The model under review builds one solid part; all positions refer to its coordinate system, in mm. Face numbers are marked on the shaded views. A direction names the side the tool comes from. Give positions to 0.01 mm unless a question says otherwise; leave off trailing zeros. Order: outer loops, then holes, each group sorted by start corner. A loop starts at its lowest first (then second) coordinate and runs counter-clockwise, first axis right, second up.
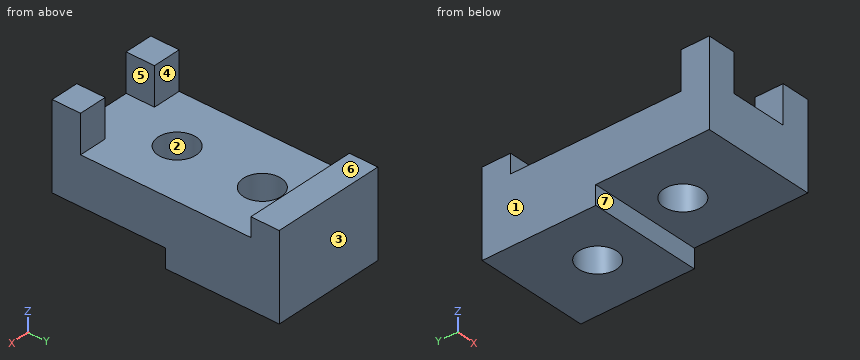
```python
from build123d import *

# Parameters (mm, degrees)
F0_W      = 60
F0_H      = 120
F1_DEPTH  = 35
F2_W      = 60
F2_H      = 15
F3_DEPTH  = 10
F4_W      = 60
F4_H      = 60
F5_DEPTH  = 10
F6_W      = 15
F6_H      = 15
F7_DEPTH  = 20
F8_W      = 15
F8_H      = 15
F9_DEPTH  = 20
F10_R     = 10
F11_DEPTH = 72.9
F12_R     = 10
F13_DEPTH = 66.7


with BuildPart() as f1:
    # F0 (on Top) → F1 (new body)
    with BuildSketch(Plane.XY):
        Rectangle(F0_W, F0_H)
    extrude(amount=F1_DEPTH)

    # F2 (on face) → F3 (join)
    with BuildSketch(Plane.XY.offset(35)):
        with Locations((0, 52.5)):
            Rectangle(F2_W, F2_H)
    extrude(amount=F3_DEPTH)

    # F4 (on face) → F5 (cut)
    with BuildSketch(Plane(origin=(0, 0, 0), x_dir=(1, 0, 0), z_dir=(0, 0, -1))):
        with Locations((0, 30)):
            Rectangle(F4_W, F4_H)
    extrude(amount=-F5_DEPTH, mode=Mode.SUBTRACT)

    # F6 (on face) → F7 (join)
    with BuildSketch(Plane.XY.offset(35)):
        with Locations((-22.5, -52.5)):
            Rectangle(F6_W, F6_H)
    extrude(amount=F7_DEPTH)

    # F8 (on face) → F9 (join)
    with BuildSketch(Plane.XY.offset(35)):
        with Locations((22.5, -52.5)):
            Rectangle(F8_W, F8_H)
    extrude(amount=F9_DEPTH)

    # F10 (on face) → F11 (cut)
    with BuildSketch(Plane.XY.offset(35)):
        with Locations((0, 25)):
            Circle(F10_R)
    extrude(amount=-F11_DEPTH, mode=Mode.SUBTRACT)

    # F12 (on face) → F13 (cut)
    with BuildSketch(Plane.XY.offset(35)):
        with Locations((0, -20)):
            Circle(F12_R)
    extrude(amount=-F13_DEPTH, mode=Mode.SUBTRACT)


solid = f1.part
```
Item 1: For line 1 (Y direction, x = 0, z = 22); line 2 (Z direction, x = 14.5, y = 38.5); line 3 (Z direction, x = 0.5, y = -1), list the stretches that pass through material, from the lowest coordinate up.
Values found:
line 1: y = -60 to -30, -10 to 15, 35 to 60
line 2: z = 0 to 35
line 3: z = 10 to 35
Item 2: For the marked faces 4, 5, 6 and 7, list the 3-axis set-ups (+Z, -Z, +X, -X, +Y, -Y) from which the entire face can be reached by the end or side of a thin tool; tool diameter is ignored.
Values found:
face 4: +Z, +X, -X
face 5: +Z, -Y
face 6: +Z, +X, -X, +Y
face 7: -Z, +X, -X, -Y
Item 3: Clearance check with flat-ended pins moving along their axes: pin 1 Ø16.5 at (x, y) = (4, 53) entering from +Z; pin 2 Ø18 at (x, y) = (-1, -19) entering from -Z; pin 3 Ø23 at (x, y) = (0, 25) entering from +Z. State where each tip first meets the part, or that it passes through.
Values found:
pin 1: stops at z = 45
pin 2: stops at z = 10
pin 3: stops at z = 35
Item 4: Take a section at A-A (y = 25). Give the boundary of the cut face in (x, z), and give its area (3 significant figures).
Values found:
outline: (-30, 0) - (-10, 0) - (-10, 35) - (-30, 35) - close; (10, 0) - (30, 0) - (30, 35) - (10, 35) - close
area: 1,400 mm2
Item 5: Take a section at D-D (z = 17). Give the boundary of the cut face in (x, y), and give its area (3 significant figures).
Values found:
outline: (-30, -60) - (30, -60) - (30, 60) - (-30, 60) - close; hole circle Ø20 at (0, -20); hole circle Ø20 at (0, 25)
area: 6,570 mm2
Item 6: Take a section at B-B (x = 0). Give the boundary of the cut face in (y, z).
Values found:
outline: (-60, 10) - (-30, 10) - (-30, 35) - (-60, 35) - close; (-10, 10) - (0, 10) - (0, 0) - (15, 0) - (15, 35) - (-10, 35) - close; (35, 0) - (60, 0) - (60, 45) - (45, 45) - (45, 35) - (35, 35) - close
Item 7: Take a section at C-C (z = 42.5). Give the boundary of the cut face in (x, y).
Values found:
outline: (-30, -60) - (-15, -60) - (-15, -45) - (-30, -45) - close; (-30, 45) - (30, 45) - (30, 60) - (-30, 60) - close; (15, -60) - (30, -60) - (30, -45) - (15, -45) - close
Item 8: Draft analysis for pull direction X (two halves, no side actions). For the marked faces 1, 2 and 3, state which applies: released by +X, released by -X, zero draft, split by the parting line, or undercut.
Values found:
face 1: released by -X
face 2: undercut
face 3: zero draft
